Model file for the job. Use its own axes, mm. Face numbers are marked on the shaded views. Round coordinates to 2 decimals unless told otherwise and drop trailing zeros. Write each loop counter-clockwise with the first axis right and the second up, starting at its lowest first coordinate (ties: lowest second). Pieces come first, ordered by that corner, then holes.
```python
from build123d import *

# Parameters (mm, degrees)
F0_R           = 5
F1_DEPTH       = 27.5
F1_DEPTH_BACK  = 27.5
F4_R           = 5
F5_DEPTH       = 55
F6_W           = 175
F6_H           = 126.1557921569
F7_DEPTH       = 12.5
F7_DEPTH_BACK  = 12.5
F8_R           = 5
F9_DEPTH       = 6.25
F9_DEPTH_BACK  = 6.25
F10_W          = 15
F10_H          = 120
F11_DEPTH      = 45
F11_DEPTH_BACK = 45
F12_R          = 5
F13_R          = 5


with BuildPart() as f1:
    # F0 (on Front) → F1 (new body, two sides)
    with BuildSketch(Plane.XZ) as f1_sk:
        with BuildLine():
            Line((-900, -10), (0, -10))
            ThreePointArc((0, -10), (10, 0), (0, 10))
            Line((0, 10), (-900, 10))
            Line((-900, 10), (-900, -10))
        make_face()
        Circle(F0_R, mode=Mode.SUBTRACT)
    extrude(amount=-F1_DEPTH)
    extrude(f1_sk.sketch, amount=F1_DEPTH_BACK)

    # F4 (on offset) → F5 (join)
    with BuildSketch(Plane.XZ.offset(27.5)):
        with BuildLine():
            Line((-10, 80), (-10, 0))
            ThreePointArc((-10, 0), (0, -10), (10, 0))
            Line((10, 0), (10, 90))
            ThreePointArc((10, 90), (7.0710678119, 97.0710678119), (0, 100))
            Line((0, 100), (-145, 100))
            Line((-145, 100), (-145, 80))
            Line((-145, 80), (-10, 80))
        make_face()
        Circle(F4_R, mode=Mode.SUBTRACT)
    extrude(amount=-F5_DEPTH)

    # F6 (on offset) → F7 (cut, two sides)
    with BuildSketch(Plane.XZ) as f7_sk:
        with Locations((-57.5, 44.8381894321)):
            Rectangle(F6_W, F6_H)
    extrude(amount=-F7_DEPTH, mode=Mode.SUBTRACT)
    extrude(f7_sk.sketch, amount=F7_DEPTH_BACK, mode=Mode.SUBTRACT)

    # F8 (on offset) → F9 (join, two sides)
    with BuildSketch(Plane.XZ) as f9_sk:
        with BuildLine():
            Line((-310, -10), (-310, -20))
            ThreePointArc((-310, -20), (-300, -30), (-290, -20))
            Line((-290, -20), (-290, -10))
            Line((-290, -10), (-300, -10))
            Line((-300, -10), (-310, -10))
        make_face()
        with Locations((-300, -20)):
            Circle(F8_R, mode=Mode.SUBTRACT)
    extrude(amount=F9_DEPTH)
    extrude(f9_sk.sketch, amount=-F9_DEPTH_BACK)

    # F10 (on offset) → F11 (join, two sides)
    with BuildSketch(Plane.XZ) as f11_sk:
        with Locations((-152.5, 70)):
            Rectangle(F10_W, F10_H)
    extrude(amount=F11_DEPTH)
    extrude(f11_sk.sketch, amount=-F11_DEPTH_BACK)

    # F12
    f12_edges = [f1.edges().sort_by_distance(p)[0] for p in [
        (-152.5, -45, 130),
        (-152.5, 45, 130),
        (-152.5, -45, 10),
        (-152.5, 45, 10),
    ]]
    fillet(f12_edges, radius=F12_R)

    # F13
    f13_edges = [f1.edges().sort_by_distance(p)[0] for p in [
        (-10, -20, 80),
        (-10, 20, 80),
    ]]
    fillet(f13_edges, radius=F13_R)


solid = f1.part
```
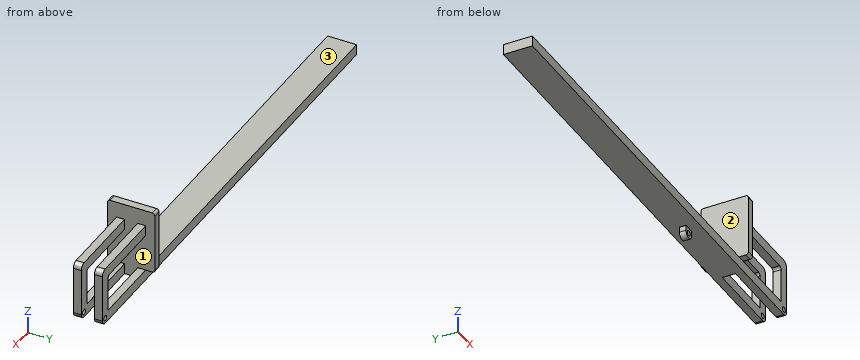
1) Pull direction Z, two halves, no side cores. Call the marked faces 1, 2 and 3: released by +Z, released by -Z, zero draft, split by the parting line, or undercut.
2) Cut at B-B on y = -20. List the corners of the cut face in (x, z), and give its area (3 significant figures).
3) Cut at C-C on x = -176. List the corners of the cut face in (y, z), and give its area (3 significant figures).
4) Cut at A-A on z = 54.5. List the corners of the cut face in (x, y).
5) Wall check: probe 1 along X at (y, z) = (-15.5, 64.5); probe 2 along Z at (x, y) = (0, 22); probe 3 along X at (y, z) = (-17, 0). Give the ranges that are in metal, low to high.
6) Flat gauge pins, fed straight in: pin 1 Ø7.5 at (y, z) = (18, 57) entering from -X; pin 2 Ø10 at (x, y) = (-152.5, 35) entering from -Z; pin 3 Ø1.5 at (y, z) = (-32.5, 49.5) entering from +X; pin 4 Ø6 at (x, z) = (0, 0) entering from -Y. Where does each tip first touch, or does it go through?
Result sheet:
1. face 1: undercut
1. face 2: zero draft
1. face 3: released by +Z
2. outline: (-900, -10) - (0, -10) arc R10 ccw to (10, 0) - (10, 90) arc R10 ccw to (0, 100) - (-145, 100) - (-145, 130) - (-160, 130) - (-160, 10) - (-900, 10) - close; hole (-145, 10) - (-10, 10) - (-10, 75) arc R5 ccw to (-15, 80) - (-145, 80) - close; hole circle Ø10 at (0, 0)
2. area: 24,400 mm2
3. outline: (-27.5, -10) - (27.5, -10) - (27.5, 10) - (-27.5, 10) - close
3. area: 1,100 mm2
4. outline: (-160, -45) - (-145, -45) - (-145, 45) - (-160, 45) - close; (-10, -27.5) - (10, -27.5) - (10, -12.5) - (-10, -12.5) - close; (-10, 12.5) - (10, 12.5) - (10, 27.5) - (-10, 27.5) - close
5. probe 1: x = -160 to -145, -10 to 10
5. probe 2: z = -10 to -5, 5 to 100
5. probe 3: x = -900 to -5, 5 to 10
6. pin 1: stops at x = -160
6. pin 2: stops at z = 10
6. pin 3: stops at x = -145
6. pin 4: passes through
